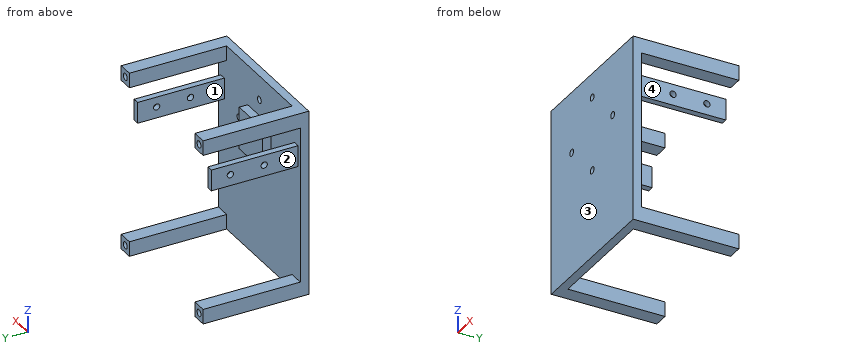
from build123d import *

# Parameters (mm, degrees)
SKETCH1_W           = 70
SKETCH1_H           = 88
BOSS_EXTRUDE1_DEPTH = 50
SKETCH2_R           = 1.65
CUT_EXTRUDE1_DEPTH  = 8
CUT_EXTRUDE2_DEPTH  = 46
SKETCH5_R           = 1.6
CUT_EXTRUDE4_DEPTH  = 73.642962495
SKETCH6_W           = 20
SKETCH6_H           = 20
BOSS_EXTRUDE2_DEPTH = 4
SKETCH7_W           = 3
SKETCH7_H           = 10
BOSS_EXTRUDE3_DEPTH = 41
SKETCH8_R           = 1.5
CUT_EXTRUDE5_DEPTH  = 10
CUT_EXTRUDE6_START  = -10
SKETCH9_R           = 1.5
CUT_EXTRUDE6_DEPTH  = 10


with BuildPart() as part:
    # Sketch1 → Boss-Extrude1 (new body)
    with BuildSketch(Plane(origin=(0, 0, 0), x_dir=(1, 0, 0), z_dir=(0, 1, 0))):
        Rectangle(SKETCH1_W, SKETCH1_H)
    extrude(amount=BOSS_EXTRUDE1_DEPTH)

    # Sketch2 → Cut-Extrude1 (cut)
    with BuildSketch(Plane(origin=(0, 50, 0), x_dir=(1, 0, 0), z_dir=(0, 1, 0))):
        with Locations(Location((-31.5, 40.5, 0), (0, 0, 270))):
            Circle(SKETCH2_R)
        with Locations(Location((31.5, 40.5, 0), (0, 0, 90))):
            Circle(SKETCH2_R)
        with Locations(Location((31.5, -40.5, 0), (0, 0, 270))):
            Circle(SKETCH2_R)
        with Locations(Location((-31.5, -40.5, 0), (0, 0, 90))):
            Circle(SKETCH2_R)
    extrude(amount=-CUT_EXTRUDE1_DEPTH, mode=Mode.SUBTRACT)

    # Sketch3 → Cut-Extrude2 (cut)
    with BuildSketch(Plane(origin=(0, 50, 0), x_dir=(1, 0, 0), z_dir=(0, 1, 0))):
        Polygon((-28, -44), (28, -44), (28, -37), (35, -37), (35, 37), (28, 37), (28, 44), (-28, 44), (-28, 37), (-35, 37), (-35, -37), (-28, -37), align=None)
    extrude(amount=-CUT_EXTRUDE2_DEPTH, mode=Mode.SUBTRACT)

    # Sketch5 → Cut-Extrude4 (cut, through all)
    with BuildSketch(Plane(origin=(0, 4, 0), x_dir=(1, 0, 0), z_dir=(0, 1, 0))):
        with Locations(Location((-17.5, -15, 0), (0, 0, 270))):
            Circle(SKETCH5_R)
        with Locations(Location((0, 2.5, 0), (0, 0, 270))):
            Circle(SKETCH5_R)
        with Locations(Location((0, -32.5, 0), (0, 0, 90))):
            Circle(SKETCH5_R)
        with Locations(Location((17.5, -15, 0), (0, 0, 90))):
            Circle(SKETCH5_R)
    extrude(amount=-CUT_EXTRUDE4_DEPTH, mode=Mode.SUBTRACT)

    # Sketch6 → Boss-Extrude2 (add)
    with BuildSketch(Plane(origin=(0, 4, 0), x_dir=(1, 0, 0), z_dir=(0, 1, 0))):
        with Locations((0, -15)):
            Rectangle(SKETCH6_W, SKETCH6_H)
    extrude(amount=BOSS_EXTRUDE2_DEPTH)

    # Sketch7 → Boss-Extrude3 (add)
    with BuildSketch(Plane(origin=(0, 4, 0), x_dir=(1, 0, 0), z_dir=(0, 1, 0))):
        with Locations((-31.5, -22.5)):
            Rectangle(SKETCH7_W, SKETCH7_H)
        with Locations((31.5, -22.5)):
            Rectangle(SKETCH7_W, SKETCH7_H)
    extrude(amount=BOSS_EXTRUDE3_DEPTH)

    # Sketch8 → Cut-Extrude5 (cut)
    with BuildSketch(Plane(origin=(-30, 0, 0), x_dir=(0, 0, -1), z_dir=(1, 0, 0))):
        with Locations((-22.75, 20)):
            Circle(SKETCH8_R)
        with Locations((-22.75, 36)):
            Circle(SKETCH8_R)
    extrude(amount=-CUT_EXTRUDE5_DEPTH, mode=Mode.SUBTRACT)

    # Sketch9 → Cut-Extrude6 (cut)
    with BuildSketch(Plane.ZY.offset(-30).offset(CUT_EXTRUDE6_START)):
        with Locations(Location((22.75, 20, 0), (0, 0, 180))):
            Circle(SKETCH9_R)
        with Locations(Location((22.75, 36, 0), (0, 0, 180))):
            Circle(SKETCH9_R)
    extrude(amount=CUT_EXTRUDE6_DEPTH, mode=Mode.SUBTRACT)


solid = part.part
CAD build for the part. Positions are in the model's coordinates, mm. Face numbers are marked on the shaded views. A direction names the side the tool comes from. Round coordinates to 2 decimals unless told otherwise and drop trailing zeros. Write each loop counter-clockwise with the first axis right and the second up, starting at its lowest first coordinate (ties: lowest second). Pieces come first, ordered by that corner, then holes. Notation, with made-up numbers: (-15, 69.25) -> (-1, 69.25) arc R18 cw to (-1, 90.25) -> close; hole circle Ø9 at (43, 53). An arc over 180 degrees is marked (long way). Answer as a JSON object with one key per item and string values.
(1) Band-saw the part on D-D, the plane z = -2.5. List the corners of the cut face in (x, y), then the cut area to 3 significant figures.
Reported:
{"outline": "(-35, 0) -> (-1.6, 0) -> (-1.6, 4) -> (-35, 4) -> close; (1.6, 0) -> (35, 0) -> (35, 4) -> (1.6, 4) -> close", "area": "267 mm^2"}
(2) Which spindle directions (+Z, -Z, +X, -X, +Y, -Y) get a long thin tool onto all of the face, cutting with end or side? Do the marked faces 1 and 2. Say none if no direction does.
Reported:
{"face 1": "+Y", "face 2": "-X, +Y"}
(3) Two-plate mould, pull along Z, no slides. Class the marked faces 3 and 4: +Z half, -Z half, draft (parallel to the pull), parting line (faces both ways), or undercut.
Reported:
{"face 3": "draft", "face 4": "undercut"}
(4) Probe probe 1 along X at (y, z) = (0.95, 15); probe 2 along Z at (x, y) = (31.1, 20); probe 3 along X at (y, z) = (47, -40.5). List the from-to ranges inside material, lowest first. Write a range as [from, to].
Reported:
{"probe 1": "x = [-35, -19.1], [-15.9, 15.9], [19.1, 35]", "probe 2": "z = [-44, -37], [17.5, 21.25], [24.25, 27.5], [37, 44]", "probe 3": "x = [-35, -33.15], [-29.85, -28], [28, 29.85], [33.15, 35]"}
(5) Pin check, flat tips, straight feed: P1, Ø2, axis at x = 3, y = 6, coming from the +Z side; P2, Ø4, axis at y = 26.5, z = 24, coming from the -X side; P3, Ø1, axis at x = 24.5, z = 20, coming from the +Y side. Stop position of each tip, or through.
Reported:
{"P1": "stops at z = 25", "P2": "stops at x = -33", "P3": "stops at y = 4"}
(6) Band-saw the part on C-C, the plane y = 43.5. Count the separate pieces of the cut face and the enclosed holes in it, then the cut area to 3 significant figures.
Reported:
{"separate pieces": "6", "enclosed holes": "4", "area": "222 mm^2"}
(7) Band-saw the part on A-A, the plane y = 6.5. List the corners of the cut face in (x, z), then the cut area to 3 significant figures.
Reported:
{"outline": "(-35, -44) -> (-28, -44) -> (-28, -37) -> (-35, -37) -> close; (-35, 37) -> (-28, 37) -> (-28, 44) -> (-35, 44) -> close; (-33, 17.5) -> (-30, 17.5) -> (-30, 27.5) -> (-33, 27.5) -> close; (-10, 5) -> (10, 5) -> (10, 25) -> (-10, 25) -> close; (28, -44) -> (35, -44) -> (35, -37) -> (28, -37) -> close; (28, 37) -> (35, 37) -> (35, 44) -> (28, 44) -> close; (30, 17.5) -> (33, 17.5) -> (33, 27.5) -> (30, 27.5) -> close", "area": "656 mm^2"}
(8) Band-saw the part on B-B, the plane x = -17.5. List the corners of the cut face in (y, z), then the cut area to 3 significant figures.
Reported:
{"outline": "(0, -44) -> (4, -44) -> (4, 13.4) -> (0, 13.4) -> close; (0, 16.6) -> (4, 16.6) -> (4, 44) -> (0, 44) -> close", "area": "339 mm^2"}
